Here's the drawing with two shaded views (mm, measured from the low corner). I have some questions. A direction names the side the tool comes from. Give positions to 0.01 mm unless a question says otherwise; leave off trailing zeros. Loops run counter-clockwise (first coordinate to the right, second up) from the corner with the lowest first, then second, coordinate; pieces in that order, holes last. Notation, with made-up numbers: (-2.75, 88.25) -> (23.25, 88.25) arc R25 ccw to (23.25, 109.25) -> close; hole circle Ø5 at (57.5, 72). An arc over 180 degrees is marked (long way). Put each result on its own line as item: value.
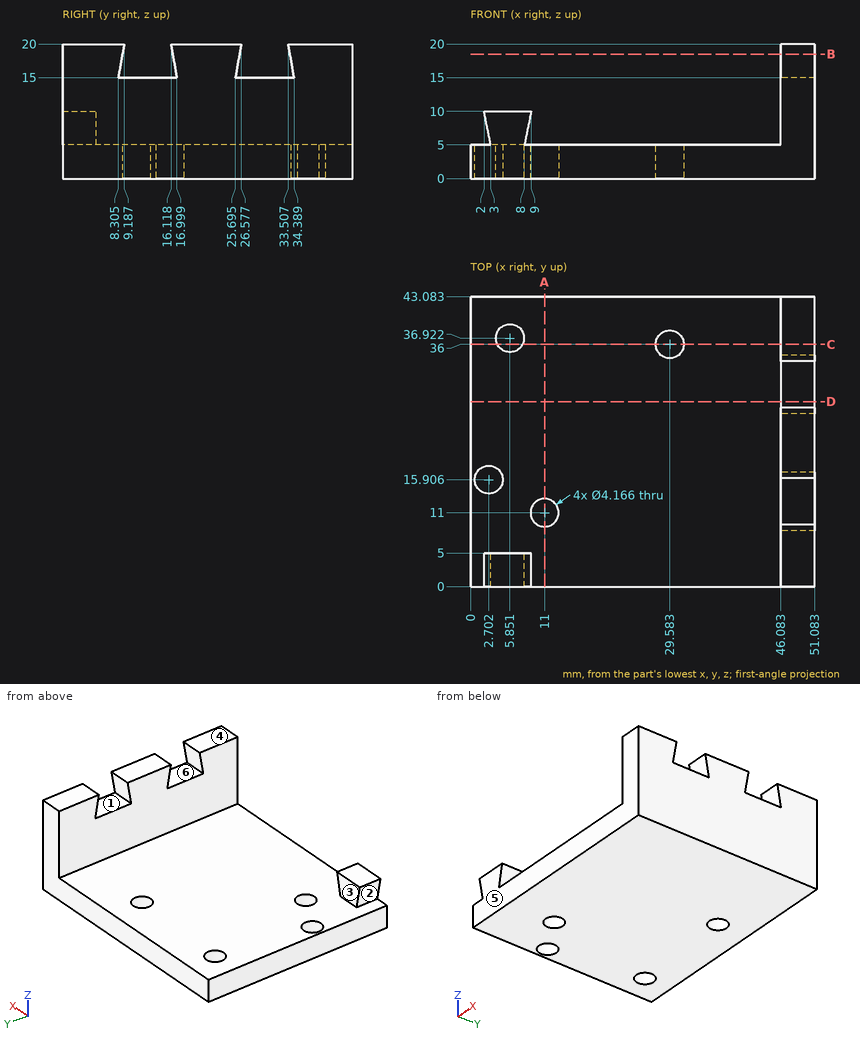
1. Thinking about a two-plate mould opening in Y: for the marked faces 4, 5 and 6, which applies, pulls with the +Y half, pulls with the -Y half, needs draft (parallel to the pull), parting line crosses it, or undercut?
Recorded:
face 4: needs draft
face 5: pulls with the -Y half
face 6: undercut
2. I need wall thicknesses on line 1 (Y direction, x = 11, z = 1.7); line 2 (Z direction, x = 40.5, y = 21); line 3 (Y direction, x = 29.5, z = 1). Which ranges of each line are inside material? Lowest first, please.
Recorded:
line 1: y = 0 to 8.92, 13.08 to 43.08
line 2: z = 0 to 5
line 3: y = 0 to 33.92, 38.08 to 43.08
3. If we section it at B-B (z = 18.5): List the corners of the cut face in (x, y) for me.
Recorded:
outline: (46.08, 0) -> (51.08, 0) -> (51.08, 8.92) -> (46.08, 8.92) -> close; (46.08, 16.38) -> (51.08, 16.38) -> (51.08, 26.31) -> (46.08, 26.31) -> close; (46.08, 33.77) -> (51.08, 33.77) -> (51.08, 43.08) -> (46.08, 43.08) -> close
4. I'm going to push flat-ended pins straight in: pin 1 (10 mm diameter, centred on x = 12.5, z = 13, fed in from +Y); pin 2 (5.5 mm diameter, centred on x = 47.5, y = 31.5, fed in from +Z); pin 3 (3.5 mm diameter, centred on x = 11, y = 11, fed in from -Z); pin 4 (6.5 mm diameter, centred on x = 5.851, y = 36.922, fed in from +Z). Where does each tip first touch, or does it pass through?
Recorded:
pin 1: stops at y = 5
pin 2: stops at z = 20
pin 3: passes through
pin 4: stops at z = 5
5. For the marked faces 1, 2 and 3, which set-ups out of +Z, -Z, +X, -X, +Y, -Y let a thin tool reach every point of the face, with its end or its side?
Recorded:
face 1: +X, -X
face 2: -X, +Y, -Y
face 3: +Z, -X, +Y
6. If we section it at D-D (y = 27.5): List the corners of the cut face in (x, z) for me.
Recorded:
outline: (0, 0) -> (51.08, 0) -> (51.08, 15) -> (46.08, 15) -> (46.08, 5) -> (0, 5) -> close
7. If we section it at C-C (y = 36): List the corners of the cut face in (x, z) for me (1 decimal), then the cut area to 3 significant figures.
Recorded:
outline: (0, 0) -> (4, 0) -> (4, 5) -> (0, 5) -> close; (7.7, 0) -> (27.5, 0) -> (27.5, 5) -> (7.7, 5) -> close; (31.7, 0) -> (51.1, 0) -> (51.1, 20) -> (46.1, 20) -> (46.1, 5) -> (31.7, 5) -> close
area: 291 mm^2
8. If we section it at A-A (x = 11): List the corners of the cut face in (y, z) for me, then the cut area to 3 significant figures.
Recorded:
outline: (0, 0) -> (8.92, 0) -> (8.92, 5) -> (0, 5) -> close; (13.08, 0) -> (43.08, 0) -> (43.08, 5) -> (13.08, 5) -> close
area: 195 mm^2
